from build123d import *

# Parameters (mm, degrees)
SKETCH_1_W          = 110
SKETCH_1_H          = 78
SKETCH_1_R          = 1.5
EXTRUDE_1_DEPTH     = 4
SKETCH_4_R          = 2
SKETCH_4_R_2        = 9.51
CUT_EXTRUDE_1_DEPTH = 68.542579163


with BuildPart() as part:
    # 草图1 → 凸台-拉伸1 (new body)
    with BuildSketch(Plane.XY):
        Rectangle(SKETCH_1_W, SKETCH_1_H)
        with Locations((-32.5, 31.5)):
            Circle(SKETCH_1_R, mode=Mode.SUBTRACT)
        with Locations((47.5, 31.5)):
            Circle(SKETCH_1_R, mode=Mode.SUBTRACT)
        with Locations((47.5, -31.5)):
            Circle(SKETCH_1_R, mode=Mode.SUBTRACT)
        with Locations((-32.5, -31.5)):
            Circle(SKETCH_1_R, mode=Mode.SUBTRACT)
    extrude(amount=EXTRUDE_1_DEPTH)

    # 草图4 → 切除-拉伸1 (cut, through all)
    with BuildSketch(Plane.XY.offset(4)):
        with Locations((-11, 17.5)):
            Circle(SKETCH_4_R)
        with Locations((-28.5, 0)):
            Circle(SKETCH_4_R)
        with Locations((-11, -17.5)):
            Circle(SKETCH_4_R)
        with Locations((6.5, 0)):
            Circle(SKETCH_4_R)
        with Locations((-11, 0)):
            Circle(SKETCH_4_R_2)
    extrude(amount=-CUT_EXTRUDE_1_DEPTH, mode=Mode.SUBTRACT)


solid = part.part
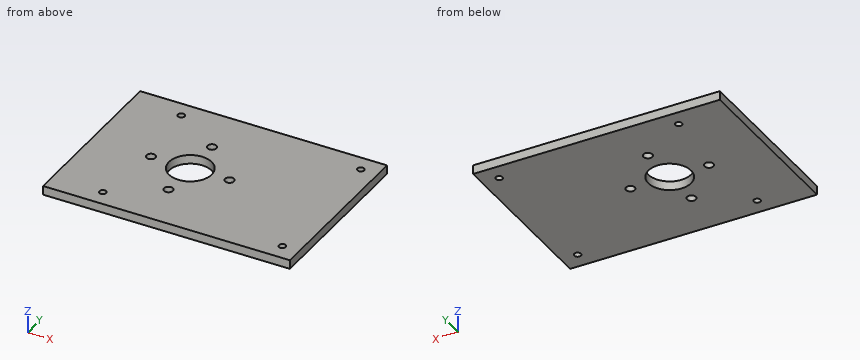
Design review of the part built by this model. Coordinates are the model's own, in mm. Coordinates: 2 decimals unless noted, no trailing zeros. Order: outer loops, then holes, each group sorted by start corner. A loop starts at its lowest first (then second) coordinate and runs counter-clockwise, first axis right, second up. Notation, with made-up numbers: (-40, -11) -> (18, -11) arc R18 ccw to (18, 16) -> close; hole circle Ø5 at (7.25, 88). An arc over 180 degrees is marked (long way). One line per item, written item: value.
1) We need section B-B, the plane y = -17.5. Give the boundary of the cut face in (x, z).
Output values:
outline: (-55, 0) -> (-13, 0) -> (-13, 4) -> (-55, 4) -> close; (-9, 0) -> (55, 0) -> (55, 4) -> (-9, 4) -> close
2) We need section D-D, the plane y = -31.5. Give the boundary of the cut face in (x, z).
Output values:
outline: (-55, 0) -> (-34, 0) -> (-34, 4) -> (-55, 4) -> close; (-31, 0) -> (46, 0) -> (46, 4) -> (-31, 4) -> close; (49, 0) -> (55, 0) -> (55, 4) -> (49, 4) -> close
3) To check wall thickness, follow probe 1 along Y at (x, z) = (-11, 1.05); probe 2 along Y at (x, z) = (47.5, 1.6); probe 3 along X at (y, z) = (32, 1.9). State the ranges of each line that lie inside material, in increasing order. Write a range as [from, to].
Output values:
probe 1: y = [-39, -19.5], [-15.5, -9.51], [9.51, 15.5], [19.5, 39]
probe 2: y = [-39, -33], [-30, 30], [33, 39]
probe 3: x = [-55, -33.91], [-31.09, 46.09], [48.91, 55]
4) We need section A-A, the plane x = 47.5. Give the boundary of the cut face in (y, z), then the cut area to 3 significant figures.
Output values:
outline: (-39, 0) -> (-33, 0) -> (-33, 4) -> (-39, 4) -> close; (-30, 0) -> (30, 0) -> (30, 4) -> (-30, 4) -> close; (33, 0) -> (39, 0) -> (39, 4) -> (33, 4) -> close
area: 288 mm2
5) Clearance check with a flat-ended pin moving along its axis: P1, Ø3, axis at x = -28.5, y = 0, coming from the -Z side. State where the tip first meets the part, or that it passes through.
Output values:
P1: passes through
6) We need section C-C, the plane z = 1. Count the separate pieces of the cut face and the enclosed holes in it, then the cut area to 3 significant figures.
Output values:
separate pieces: 1
enclosed holes: 9
area: 8,220 mm2
